Here's how the part is built. I have some questions about the finished solid (model axes, mm). Face numbers are marked on the shaded views. A direction names the side the tool comes from. Round coordinates to 2 decimals unless told otherwise and drop trailing zeros. Write each loop counter-clockwise with the first axis right and the second up, starting at its lowest first coordinate (ties: lowest second). Pieces come first, ordered by that corner, then holes. Notation, with made-up numbers: (75.5, -27) -> (105.5, -27) arc R34 ccw to (105.5, 4) -> close; hole circle Ø8 at (0, -26.75). An arc over 180 degrees is marked (long way). Answer in a Markdown table with one row per item. Add a question column.
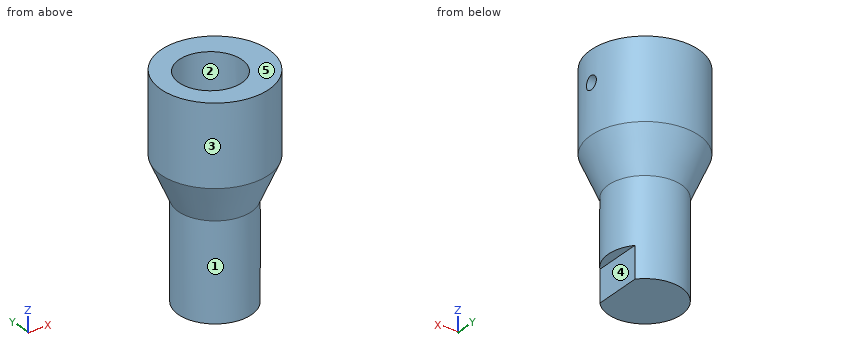
from build123d import *

# Parameters (mm, degrees)
IZIM2_W               = 1.58
IZIM2_H               = 5.56
KES_EKSTR_ZYON1_DEPTH = 5
IZIM6_R               = 5.555
KES_EKSTR_ZYON2_DEPTH = 14.06
IZIM9_R               = 1.19
KES_EKSTR_ZYON3_DEPTH = 14.06


with BuildPart() as part:
    # Çizim1 → Döndür2 (revolve)
    with BuildSketch(Plane(origin=(0, 0, 0), x_dir=(0, 0, -1), z_dir=(1, 0, 0)), mode=Mode.PRIVATE) as d_nd_r2_sk:
        Polygon((-16.346129032, 9.525), (-2.286129032, 9.525), (4.813870968, 6.45), (21.753870968, 6.45), (21.753870968, 0), (-16.346129032, 0), align=None)
    revolve(d_nd_r2_sk.sketch.rotate(Axis((0, 0, 16.346129032), (0, 0, -1)), 90), axis=Axis((0, 0, 16.346129032), (0, 0, -1)))

    # Çizim2 → Kes-Ekstrüzyon1 (cut, symmetric)
    with BuildSketch(Plane(origin=(0, 0, 0), x_dir=(1, 0, 0), z_dir=(0, 1, 0))):
        with Locations((5.66, 18.973870968)):
            Rectangle(IZIM2_W, IZIM2_H)
    extrude(amount=KES_EKSTR_ZYON1_DEPTH, both=True, mode=Mode.SUBTRACT)

    # Çizim6 → Kes-Ekstrüzyon2 (cut)
    with BuildSketch(Plane.XY.offset(16.346129032)):
        with Locations((-0.796682274, 0)):
            Circle(IZIM6_R)
    extrude(amount=-KES_EKSTR_ZYON2_DEPTH, mode=Mode.SUBTRACT)

    # Çizim9 → Kes-Ekstrüzyon3 (cut)
    with BuildSketch(Plane(origin=(0, 0, 0), x_dir=(0, 0, -1), z_dir=(1, 0, 0))):
        with Locations(Location((-10.918037958, 0, 0), (0, 0, 180))):
            Circle(IZIM9_R)
    extrude(amount=KES_EKSTR_ZYON3_DEPTH, mode=Mode.SUBTRACT)


solid = part.part
Item 1: If we section it at C-C on z = -11: Please give me the cut outline in (x, y), then the cut area to 3 significant figures.
Item 2: I need wall thicknesses on line 1 along Z through (x, y) = (-4.75, 2); line 2 along Y through (x, z) = (2.5, 11); line 3 along X through (y, z) = (-1.5, 11.5). Which ranges of each line are inside material? Lowest first, please. Write a range as from..to.
Item 3: If we section it at B-B on z = 13: Please give me the cut outline in (x, y) (3 decimals), then the cut area to 3 significant figures.
Item 4: For P1, Ø0.8, axis at x = 6, y = 2, coming from the -Z side; P2, Ø2, axis at x = 7.5, y = 5, coming from the -Z side; P3, Ø5, axis at y = 1, z = -8, coming from the -X side, each with a flat end and sliding along its axis, tell me the tip position at first contact or that it passes through.
Item 5: If we section it at D-D on x = 0: Please give me the cut outline in (y, z) (3 decimals), then the cut area to 3 significant figures.
Item 6: On a 3-axis mill with a long thin cutter (end or side, diameter ignored), from which of +Z, -Z, +X, -X, +Y, -Y can I reach the whole of each face in a straight line? I mean the marked faces 1, 2, 3, 4 and 5. Say none if no direction works.
Item 7: If we section it at A-A on y = 0: Please give me the cut outline in (x, z) (3 decimals), then the cut area to 3 significant figures.
Results list:
| question | item | result |
|---|---|---|
| 1 | outline | circle Ø12.9 at (0, 0) |
| 1 | area | 131 mm² |
| 2 | line 1 | -21.75..2.29 |
| 2 | line 2 | -9.19..-4.47, 4.47..9.19 |
| 2 | line 3 | -9.41..-6.15, 4.55..9.41 |
| 3 | outline | circle Ø19.05 at (0, 0); hole circle Ø11.11 at (-0.797, 0) |
| 3 | area | 188 mm² |
| 4 | P1 | z = -16.19 |
| 4 | P2 | z = -1.2 |
| 4 | P3 | x = -6.45 |
| 5 | outline | (-9.525, 2.286) -> (-6.45, -4.814) -> (-6.45, -21.754) -> (6.45, -21.754) -> (6.45, -4.814) -> (9.525, 2.286) -> (9.525, 16.346) -> (5.498, 16.346) -> (5.498, 2.286) -> (-5.498, 2.286) -> (-5.498, 16.346) -> (-9.525, 16.346) -> close |
| 5 | area | 445 mm² |
| 6 | face 1 | -Z |
| 6 | face 2 | +Z |
| 6 | face 3 | +Z, -Z |
| 6 | face 4 | -Z, +X, +Y, -Y |
| 6 | face 5 | +Z, +X, -X, +Y, -Y |
| 7 | outline | (-9.525, 2.286) -> (-6.45, -4.814) -> (-6.45, -21.754) -> (4.87, -21.754) -> (4.87, -16.194) -> (6.45, -16.194) -> (6.45, -4.814) -> (9.525, 2.286) -> (9.525, 9.728) -> (4.758, 9.728) -> (4.758, 2.286) -> (-6.352, 2.286) -> (-6.352, 16.346) -> (-9.525, 16.346) -> close; (4.758, 12.108) -> (9.525, 12.108) -> (9.525, 16.346) -> (4.758, 16.346) -> close |
| 7 | area | 423 mm² |
